For this review, take the finished solid that the model builds, in its own axes (mm). A direction names the side the tool comes from. Coordinates: 2 decimals unless noted, no trailing zeros. Order: outer loops, then holes, each group sorted by start corner. A loop starts at its lowest first (then second) coordinate and runs counter-clockwise, first axis right, second up. Notation, with made-up numbers: M 8.25,-39.75 L 19.25,-39.75 A22 cw 19.25,-1.75 Z; hole C 48,18.5 d6. An arc over 180 degrees is marked long. Use CSV: the item, a comma, the result in double quotes.
```python
from build123d import *

# Parameters (mm, degrees)
SKETCH1_R           = 300
SKETCH1_R_2         = 150
BOSS_EXTRUDE1_DEPTH = 400
BOSS_EXTRUDE2_DEPTH = 300
SKETCH6_R           = 100
CUT_EXTRUDE1_DEPTH  = 951


with BuildPart() as part:
    # Sketch1 → Boss-Extrude1 (new body, symmetric)
    with BuildSketch(Plane.XY):
        Circle(SKETCH1_R)
        Circle(SKETCH1_R_2, mode=Mode.SUBTRACT)
    extrude(amount=BOSS_EXTRUDE1_DEPTH, both=True)

    # Sketch2 → Boss-Extrude2 (add, symmetric)
    with BuildSketch(Plane.XY):
        with BuildLine():
            Line((0, 300), (0, 650))
            Line((0, 650), (400, 650))
            Line((400, 650), (400, 450))
            Line((400, 450), (200, 450))
            Line((200, 450), (200, 223.60679775))
            ThreePointArc((200, 223.60679775), (107.046626932, 280.251707689), (0, 300))
        make_face()
    extrude(amount=BOSS_EXTRUDE2_DEPTH, both=True)

    # Sketch5 → Revolve1 (revolve)
    with BuildSketch(Plane.XY, mode=Mode.PRIVATE) as revolve1_sk:
        Polygon((500, 1050), (500, 450), (700, 450), (700, 650), (600, 1050), align=None)
    revolve(revolve1_sk.sketch.rotate(Axis((400, 1046.547462699, 0), (0, -1, 0)), 180), axis=Axis((400, 1046.547462699, 0), (0, -1, 0)))  # turned: the seam where the file's is

    # Sketch6 → Cut-Extrude1 (cut, through all)
    with BuildSketch(Plane(origin=(0, 650, 0), x_dir=(1, 0, 0), z_dir=(0, 1, 0))):
        with Locations(Location((400, 0, 0), (0, 0, 180))):  # turned: the seam where the file's is
            Circle(SKETCH6_R)
    extrude(amount=-CUT_EXTRUDE1_DEPTH, mode=Mode.SUBTRACT)


solid = part.part
```
Item 1: To check wall thickness, follow line 1 along Z through (x, y) = (400, 582); line 2 along Z through (x, y) = (400, 712.5) (3 decimals); line 3 along X through (y, z) = (355, -178). State the ranges of each line that lie inside material, in increasing order. Write a range as [from, to].
Solutions:
line 1,"[-300, -100], [100, 300]"
line 2,"[-284.375, -100], [100, 284.375]"
line 3,"[0, 200]"
Item 2: Draft analysis for pull direction Z (two halves, no side actions). For faces 1 (the face through (473.704, 745.8, -67.585)), 2 (the face through (62, 138, 400)), 3 (the face through (200, 338, 4)), state which applies: released by +Z, released by -Z, zero draft, split by the parting line, or undercut.
Solutions:
face 1,"undercut"
face 2,"released by +Z"
face 3,"zero draft"
Item 3: For faces 4 (the face through (502, 450, -4)), 5 (the face through (-19.527, 148.724, -5.6)), 6 (the face through (0, 473, 4)), 7 (the face through (64, 650, 4)), list the 3-axis set-ups (+Z, -Z, +X, -X, +Y, -Y) from which the entire face can be reached by the end or side of a thin tool; tool diameter is ignored.
Solutions:
face 4,"+Z, -Z, +X"
face 5,"+Z, -Z"
face 6,"+Z, -Z, -X, +Y"
face 7,"-X, +Y"
Item 4: Add section B-B on x = -49. State the section outline as (y, z) points, and give its area (3 significant figures).
Solutions:
outline,"M -295.97,-400 L -141.77,-400 L -141.77,400 L -295.97,400 Z; M 141.77,-400 L 295.97,-400 L 295.97,400 L 141.77,400 Z"
area,"247,000 mm^2"
Item 5: Clearance check with flat-ended pins moving along their axes: pin 1 Ø12 at (y, z) = (668, -160) entering from +X; pin 2 Ø1 at (x, z) = (-174.5, -290.5) entering from -Y; pin 3 Ø3 at (x, y) = (430, 826) entering from +Z. State where each tip first meets the part, or that it passes through.
Solutions:
pin 1,"x = 652.6"
pin 2,"y = -244.38"
pin 3,"z = 254.65"
Item 6: Add section C-C on y = 104. State the section outline as (x, z) points, and give its area (3 significant figures).
Solutions:
outline,"M -281.4,-400 L -108.09,-400 L -108.09,400 L -281.4,400 Z; M 108.09,-400 L 281.4,-400 L 281.4,400 L 108.09,400 Z"
area,"277,000 mm^2"
Item 7: Add section D-D on y = 329. State the section outline as (x, z) points, and give its area (3 significant figures).
Solutions:
outline,"M 0,-300 L 200,-300 L 200,300 L 0,300 Z"
area,"120,000 mm^2"
Item 8: Add section A-A on z = 0. State the section outline as (x, y) points, and give its area (3 significant figures).
Solutions:
outline,"M 0,300 A300 ccw long 200,223.61 L 200,450 L 300,450 L 300,1050 L 200,1050 L 100,650 L 0,650 Z; M 500,450 L 700,450 L 700,650 L 600,1050 L 500,1050 Z; hole C 0,0 d300"
area,"467,000 mm^2"
